```python
from build123d import *

# Parameters (mm, degrees)
ESQUISSE1_R                  = 49
EXTRUSION1_DEPTH             = 1
ENL_V_MAT_EXTRU_1_DEPTH      = 2
R_P_TITION_CIRCULAIRE1_COUNT = 24
ESQUISSE3_R                  = 21
EXTRUSION2_DEPTH             = 2.125
ESQUISSE4_R                  = 16
ENL_V_MAT_EXTRU_2_DEPTH      = 3.125
ENL_V_MAT_EXTRU_2_DEPTH_BACK = 3.125
CHANFREIN1_SIZE              = 0.5


with BuildPart() as part:
    # Esquisse1 → Extrusion1 (new body, symmetric)
    with BuildSketch(Plane.XY):
        Circle(ESQUISSE1_R)
    extrude(amount=EXTRUSION1_DEPTH, both=True)

    # Esquisse2 → Enlèv. mat.-Extru.1 (cut, symmetric)
    with BuildSketch(Plane.XY):
        with BuildLine():
            Line((-5.376168106, 48.704176582), (-3.276608177, 45.705694255))
            ThreePointArc((-3.276608177, 45.705694255), (1.042685581, 44.138289656), (3.986086914, 47.666666667))
            Line((3.986086914, 47.666666667), (4.083333333, 48.829564701))
            ThreePointArc((4.083333333, 48.829564701), (-0.649450523, 48.995695872), (-5.376168106, 48.704176582))
        make_face()
    enl_v_mat_extru_1 = extrude(amount=ENL_V_MAT_EXTRU_1_DEPTH, both=True, mode=Mode.SUBTRACT)

    # Répétition circulaire1: Enlèv. mat.-Extru.1 ×24 about axis
    r_p_tition_circulaire1_axis = Axis((0, 0, 0), (0, 0, 1))
    for i in range(1, R_P_TITION_CIRCULAIRE1_COUNT):
        add(enl_v_mat_extru_1.rotate(r_p_tition_circulaire1_axis, i * 360 / R_P_TITION_CIRCULAIRE1_COUNT), mode=Mode.SUBTRACT)

    # Esquisse3 → Extrusion2 (add, symmetric)
    with BuildSketch(Plane.XY):
        Circle(ESQUISSE3_R)
    extrude(amount=EXTRUSION2_DEPTH, both=True)

    # Esquisse4 → Enlèv. mat.-Extru.2 (cut, two sides)
    with BuildSketch(Plane.XY) as enl_v_mat_extru_2_sk:
        Circle(ESQUISSE4_R)
    extrude(amount=ENL_V_MAT_EXTRU_2_DEPTH, mode=Mode.SUBTRACT)
    extrude(enl_v_mat_extru_2_sk.sketch, amount=-ENL_V_MAT_EXTRU_2_DEPTH_BACK, mode=Mode.SUBTRACT)

    # Chanfrein1
    chanfrein1_edges = [part.edges().sort_by_distance(p)[0] for p in [
        (-21, 0, -2.125),
        (-21, 0, 2.125),
        (-16, 0, -2.125),
        (-16, 0, 2.125),
    ]]
    chamfer(chanfrein1_edges, length=CHANFREIN1_SIZE)


solid = part.part
```
Verification items for the finished model (mm, model axes). A direction names the side the tool comes from. Give positions to 0.01 mm unless a question says otherwise; leave off trailing zeros. Loops run counter-clockwise (first coordinate to the right, second up) from the corner with the lowest first, then second, coordinate; pieces in that order, holes last.
1. Set-up check for faces 4 (the flat face through (47.226, 4.341, 0.014)), 5 (the flat face through (-47.226, -4.341, 0.014)), 6 (the cylindrical face through (42.87, 10.48, 0.01)), 7 (the cylindrical face through (-38.49, -30.323, 0.014)), 8 (the flat face through (-4.341, 47.226, 0.014)): record each of +Z, -Z, +X, -X, +Y, -Y from which the full face is reachable in a straight line by a thin tool's end or side.
2. Thickness scan on line 1 (Y direction, x = 0, z = -0.85); line 2 (Z direction, x = 20.5, y = -10). Record the ranges inside material, lowest first.
3. Go/stop test with flat-tipped pins: pin 1 Ø1 at (y, z) = (-30, 0.5) entering from +X; pin 2 Ø1.5 at (x, y) = (2, -22.5) entering from -Z; pin 3 Ø8 at (x, y) = (-11.5, 4.5) entering from -Z. Record where each tip stops, or that it passes through.
4. Mould release check, pull along Y, two halves, no side actions. Record for faces 1 (the cylindrical face through (38.49, 30.323, 0.014)), 2 (the cylindrical face through (37.72, -22.91, 0.01)), 3 (the cylindrical face through (30.323, -38.49, 0.014)): released by +Y, released by -Y, zero draft, split by the parting line, or undercut.
5. Section check C-C, the plane y = 23.5. Enter the section's corners in (x, z).
6. Section check A-A, the plane y = 0. Enter the section's corners in (x, z) (3 decimals).
Geometry says:
1. face 4: +Z, -Z, +X
1. face 5: +Z, -Z, -X
1. face 6: +Z, -Z
1. face 7: +Z, -Z, -X, -Y
1. face 8: +Z, -Z, +Y
2. line 1: y = -44 to -16, 16 to 44
2. line 2: z = -1 to 1
3. pin 1: stops at x = 39.12
3. pin 2: stops at z = -1
3. pin 3: stops at z = -1.97
4. face 1: released by +Y
4. face 2: undercut
4. face 3: released by -Y
5. outline: (-37.6, -1) - (37.6, -1) - (37.6, 1) - (-37.6, 1) - close
6. outline: (-44, -1) - (-21, -1) - (-21, -1.625) - (-20.5, -2.125) - (-16.5, -2.125) - (-16, -1.625) - (-16, 1.625) - (-16.5, 2.125) - (-20.5, 2.125) - (-21, 1.625) - (-21, 1) - (-44, 1) - close; (16, -1.625) - (16.5, -2.125) - (20.5, -2.125) - (21, -1.625) - (21, -1) - (44, -1) - (44, 1) - (21, 1) - (21, 1.625) - (20.5, 2.125) - (16.5, 2.125) - (16, 1.625) - close
